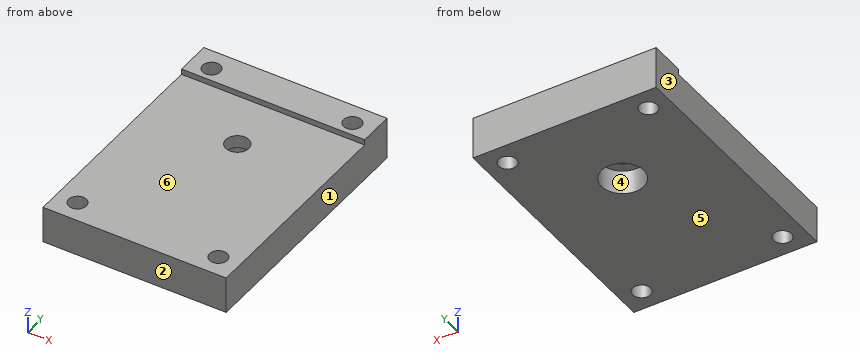
Autodesk Inventor part; units mm, degrees
ref_plane "YZ Plane" through (0, 0, 0) normal (1, 0, 0) x (0, 1, 0)
ref_plane "XZ Plane" through (0, 0, 0) normal (0, 1, 0) x (-1, 0, 0)
ref_plane "XY Plane" through (0, 0, 0) normal (0, 0, 1) x (1, 0, 0)
sketch "Sketch1" plane through (0, 0, 0) normal (0, 0, 1) x (1, 0, 0)
  line L0 (-45.5, 0) -> (45.5, 0) construction
  line L1 (0, -75.5) -> (0, 50.5) construction
  line L2 (-32.5, 32.5) -> (32.5, 32.5)
  line L3 (32.5, 32.5) -> (32.5, -57.5)
  line L4 (32.5, -57.5) -> (-32.5, -57.5)
  line L5 (-32.5, -57.5) -> (-32.5, 32.5)
  point P0 (0, 0)
  point P1 (0, 32.5)
  point P2 (32.5, -12.5)
  dimension "d0" = 65
  dimension "d28" = 32.5
  dimension "d29" = 57.5
extrude "Extrusion1" add sketch "Sketch1" along normal blind 15
sketch "Sketch2" plane through (0, 0, 0) normal (0, 0, -1) x (-1, 0, 0)
  point P0 (0, 0)
hole "Hole1" at (0, 0, 0) direction (0, 0, 1) diameter 8.2 end through all counterbore diameter 15 counterbore depth 8.5
sketch "Sketch3" plane through (0, 0, 15) normal (0, 0, 1) x (1, 0, 0)
  line L0 (-45.5, 0) -> (45.5, 0)
  line L1 (0, -75.5) -> (0, 50.5)
  point P0 (0, 0)
  point P1 (-25, 25)
  dimension "d16" = 25
  dimension "d17" = 25
hole "Hole2" at (-25, 25, 15) direction (0, 0, -1) diameter 6.3 end through all
pattern_linear "Rectangular Pattern2" count 2 spacing 50 along (1, 0, 0) count 2 spacing 75 along (0, -1, 0) of "Hole2"
sketch "Sketch4" plane through (0, 0, 15) normal (0, 0, 1) x (1, 0, 0)
  circle A0 centre (0, 0) radius 4.1 construction
  line L0 (32.5, 32.5) -> (32.5, -57.5) construction
  line L1 (32.5, -57.5) -> (-32.5, -57.5) construction
  line L2 (-32.5, -57.5) -> (-32.5, 32.5) construction
  line L3 (-32.5, 32.5) -> (32.5, 32.5) construction
  line L4 (-32.5, -57.5) -> (32.5, -57.5)
  line L5 (32.5, -57.5) -> (32.5, 20)
  line L6 (32.5, 20) -> (-32.5, 20)
  line L7 (-32.5, 20) -> (-32.5, -57.5)
  circle A1 centre (25, -50) radius 3.15
  circle A2 centre (-25, -50) radius 3.15
  circle A3 centre (25, 25) radius 3.15
  circle A4 centre (-25, 25) radius 3.15
  dimension "d42" = 20
extrude "Extrusion2" cut sketch "Sketch4" against normal blind 2 contours L7 L6 L5 L4 | A1 | A2
properties part number "P101" material "Aluminium"
The model under review builds one solid part; all positions refer to its coordinate system, in mm. Face numbers are marked on the shaded views. A direction names the side the tool comes from. Give positions to 0.01 mm unless a question says otherwise; leave off trailing zeros. Write each loop counter-clockwise with the first axis right and the second up, starting at its lowest first coordinate (ties: lowest second). Pieces come first, ordered by that corner, then holes.
(1) Consider section C-C, the plane x = 0. Give the boundary of the cut face in (y, z), and give its area (3 significant figures).
(2) The part is to be moulded in two halves that separate along X. For the marked faces 1, 2, 3 and 4, say which applies: released by +X, released by -X, zero draft, split by the parting line, or undercut.
(3) For P1, Ø1, axis at x = 14, z = 14, coming from the -Y side; P2, Ø7, axis at x = 25, y = -50, coming from the +Z side; P3, Ø7.5, axis at x = -1, y = 3.5, coming from the -Z side, all flat-tipped, find the tip position at first contact; note any pin that passes through.
(4) Consider section A-A, the plane y = -50. Give the boundary of the cut face in (x, z).
(5) Tool access review of the marked faces 5 and 6: name each direction out of +Z, -Z, +X, -X, +Y, -Y from which nothing blocks a thin tool from reaching the whole face with its end or side.
(6) To check wall thickness, follow L1, parallel to Y at x = -25, z = 7.75; L2, parallel to X at y = -50, z = 7.75; L3, parallel to Y at x = 0, z = 11.55. State the ranges of each line that lie inside material, in increasing order.
(7) Consider section D-D, the plane z = 10.75. Give the boundary of the cut face in (x, y), and give its area (3 significant figures).
(8) Consider section B-B, the plane x = -25. Give the boundary of the cut face in (y, z), and give its area (3 significant figures).
Returned:
1. outline: (-57.5, 0) - (-7.5, 0) - (-7.5, 8.5) - (-4.1, 8.5) - (-4.1, 13) - (-57.5, 13) - close; (4.1, 8.5) - (7.5, 8.5) - (7.5, 0) - (32.5, 0) - (32.5, 15) - (20, 15) - (20, 13) - (4.1, 13) - close
1. area: 1,030 mm2
2. face 1: released by +X
2. face 2: zero draft
2. face 3: released by -X
2. face 4: undercut
3. P1: stops at y = 20
3. P2: stops at z = 13
3. P3: stops at z = 8.5
4. outline: (-32.5, 0) - (-28.15, 0) - (-28.15, 13) - (-32.5, 13) - close; (-21.85, 0) - (21.85, 0) - (21.85, 13) - (-21.85, 13) - close; (28.15, 0) - (32.5, 0) - (32.5, 13) - (28.15, 13) - close
5. face 5: -Z, +X, -X, +Y, -Y
5. face 6: +Z, +X, -X, -Y
6. L1: y = -57.5 to -53.15, -46.85 to 21.85, 28.15 to 32.5
6. L2: x = -32.5 to -28.15, -21.85 to 21.85, 28.15 to 32.5
6. L3: y = -57.5 to -4.1, 4.1 to 32.5
7. outline: (-32.5, -57.5) - (32.5, -57.5) - (32.5, 32.5) - (-32.5, 32.5) - close; hole circle Ø6.3 at (-25, -50); hole circle Ø6.3 at (-25, 25); hole circle Ø8.2 at (0, 0); hole circle Ø6.3 at (25, -50); hole circle Ø6.3 at (25, 25)
7. area: 5,670 mm2
8. outline: (-57.5, 0) - (-53.15, 0) - (-53.15, 13) - (-57.5, 13) - close; (-46.85, 0) - (21.85, 0) - (21.85, 15) - (20, 15) - (20, 13) - (-46.85, 13) - close; (28.15, 0) - (32.5, 0) - (32.5, 15) - (28.15, 15) - close
8. area: 1,020 mm2
